from build123d import *

# Parameters (mm, degrees)
SKETCH1_R           = 20
BOSS_EXTRUDE1_DEPTH = 5
BOSS_EXTRUDE2_DEPTH = 4


with BuildPart() as part:
    # Sketch1 → Boss-Extrude1 (new body)
    # profile 1 of 4: a face of its own
    with BuildSketch(Plane.XY):
        with BuildLine():
            Line((0, 14.047165148), (0, 20.609217456))
            add(Edge.make_bspline(
                [(0, 20.609217456), (-5.5, 20.609217456), (-11, 24.303121583)],
                knots=[0.5, 0.5, 0.5, 1, 1, 1], degree=2))
            add(Edge.make_bspline(
                [(-11, 24.303121583), (-25.025952509, 37.034801988), (-53.805838246, 39.750693097), (-64, 20.609217456)],
                knots=[0, 0, 0, 0, 1, 1, 1, 1], degree=3))
            Line((-64, 20.609217456), (-62.236730193, 10.609217456))
            Line((-62.236730193, 10.609217456), (-59.055336952, -7.433360194))
            ThreePointArc((-59.055336952, -7.433360194), (-55.635135519, -13.357322848), (-49.207259422, -15.696878417))
            Line((-49.207259422, -15.696878417), (-31.207259422, -15.696878417))
            ThreePointArc((-31.207259422, -15.696878417), (-26.207259422, -14.357132455), (-22.547005384, -10.696878417))
            Line((-22.547005384, -10.696878417), (-13.886751346, 4.303121583))
            ThreePointArc((-13.886751346, 4.303121583), (-13.219249284, 5.312773474), (-12.434656927, 6.234386612))
            add(Edge.make_bspline(
                [(-12.434656927, 6.234386612), (-6.217328463, 14.047165148), (0, 14.047165148)],
                knots=[0.052283446, 0.052283446, 0.052283446, 0.5, 0.5, 0.5], degree=2))
        make_face()
        with Locations((-38, 9.303121583)):
            Circle(SKETCH1_R, mode=Mode.SUBTRACT)
    # profile 2 of 4: a face of its own
    with BuildSketch(Plane.XY):
        with BuildLine():
            add(Edge.make_bspline(
                [(11, 24.303121583), (5.5, 20.609217456), (0, 20.609217456)],
                knots=[0, 0, 0, 0.5, 0.5, 0.5], degree=2))
            Line((0, 20.609217456), (0, 14.047165148))
            add(Edge.make_bspline(
                [(0, 14.047165148), (6.217328463, 14.047165148), (12.434656927, 6.234386612)],
                knots=[0.5, 0.5, 0.5, 0.947716554, 0.947716554, 0.947716554], degree=2))
            ThreePointArc((12.434656927, 6.234386612), (13.219249284, 5.312773474), (13.886751346, 4.303121583))
            Line((13.886751346, 4.303121583), (22.547005384, -10.696878417))
            ThreePointArc((22.547005384, -10.696878417), (26.207259422, -14.357132455), (31.207259422, -15.696878417))
            Line((31.207259422, -15.696878417), (49.207259422, -15.696878417))
            ThreePointArc((49.207259422, -15.696878417), (55.635135519, -13.357322848), (59.055336952, -7.433360194))
            Line((59.055336952, -7.433360194), (62.236730193, 10.609217456))
            Line((62.236730193, 10.609217456), (64, 20.609217456))
            add(Edge.make_bspline(
                [(11, 24.303121583), (25.025952509, 37.034801988), (53.805838246, 39.750693097), (64, 20.609217456)],
                knots=[0, 0, 0, 0, 1, 1, 1, 1], degree=3))
        make_face()
        with Locations((38, 9.303121583)):
            Circle(SKETCH1_R, mode=Mode.SUBTRACT)
    # profile 3 of 4: a face of its own
    with BuildSketch(Plane.XY):
        Polygon((64, 10.609217456), (64, 20.609217456), (62.236730193, 10.609217456), align=None)
    # profile 4 of 4: a face of its own
    with BuildSketch(Plane.XY):
        Polygon((-62.236730193, 10.609217456), (-64, 20.609217456), (-64, 10.609217456), align=None)
    extrude(amount=BOSS_EXTRUDE1_DEPTH)

    # Sketch3 → Boss-Extrude2 (add)
    with BuildSketch(Plane.ZY.offset(64)):
        with BuildLine():
            Line((5, 20.609217456), (124.102313443, -0.391733869))
            ThreePointArc((124.102313443, -0.391733869), (131.571415965, -2.746732848), (138.176496403, -6.954633166))
            Line((138.176496403, -6.954633166), (153.084888892, -19.464259805))
            ThreePointArc((153.084888892, -19.464259805), (153.968406613, -21.161481556), (153.393030976, -22.986339937))
            Line((153.393030976, -22.986339937), (151.786061952, -24.901451044))
            ThreePointArc((151.786061952, -24.901451044), (150.088840201, -25.784968765), (148.26398182, -25.209593128))
            Line((148.26398182, -25.209593128), (134.895046755, -13.991724646))
            ThreePointArc((134.895046755, -13.991724646), (128.289966317, -9.783824329), (120.820863794, -7.428825349))
            Line((120.820863794, -7.428825349), (5, 12.993517867))
            Line((5, 12.993517867), (5, 10.609217456))
            Line((5, 10.609217456), (0, 10.609217456))
            Line((0, 10.609217456), (0, 20.609217456))
            Line((0, 20.609217456), (5, 20.609217456))
        make_face()
    boss_extrude2 = extrude(amount=-BOSS_EXTRUDE2_DEPTH)

    # Mirror1: Boss-Extrude2 across plane
    add(boss_extrude2.mirror(Plane(origin=(0, 0, 0), x_dir=(0, 0, 1), z_dir=(1, 0, 0))))


solid = part.part
Source: CAD feature listing. Evaluate the final solid. Frame: model axes, mm. A direction names the side the tool comes from. Give positions to 0.01 mm unless a question says otherwise; leave off trailing zeros. Write each loop counter-clockwise with the first axis right and the second up, starting at its lowest first coordinate (ties: lowest second). Pieces come first, ordered by that corner, then holes. Notation, with made-up numbers: (-22.5, 63.25) - (29.5, 63.25) arc R31 ccw to (29.5, 94.25) - close; hole circle Ø2 at (29.25, 31.5). An arc over 180 degrees is marked (long way). Write item = value, one per line. Start each with the question number.
Q1. Pin query (flat end, axial travel): pin 1 Ø0.5 at (x, z) = (63.5, 2) entering from -Y; pin 2 Ø12 at (x, y) = (22.5, 26) entering from +Z; pin 3 Ø2.5 at (x, z) = (-38, 3.5) entering from -Y. Return the tip coordinate at first contact, or that it passes through.
Q2. Reachability of faces 4 (the cylindrical face through (-26.271, -14.394, 2.465)), 5 (the flat face through (60.624, 1.462, 2.465)), 6 (the flat face through (-62.03, 2.64, 63.72)) from +Z, -Z, +X, -X, +Y, -Y: full face, straight path, thin tool, end or side. Return the list, or none.
Q3. Cut plane A-A, the plane z = 132. Return loops of the section in (x, y), then the cut area to 3 significant figures.
Q4. Draft query along X for faces 1 (the cylindrical face through (26.14, -14.32, 2.46)), 2 (the flat face through (62, -13.1, 145.5)), 3 (the flat face through (64, 3, 77)). Return one class per face: +X half, -X half, draft (parallel to the pull), parting line (faces both ways), or undercut.
Q5. Cut plane B-B, the plane z = 67.5. Return loops of the section in (x, y), then the cut area to 3 significant figures.
Q6. Material intervals for probe 1 along Y at (x, z) = (-38, 2.2); probe 2 along X at (y, z) = (19, 13); probe 3 along Z at (x, y) = (55, 26.5), sorted ascending.
Computed values:
q1.pin_1 = 10.61
q1.pin_2 = 5
q1.pin_3 = -15.7
q2.face_4 = +Z, -Z, -Y
q2.face_5 = -Z, +X, -Y
q2.face_6 = +X, -X, -Y
q3.outline = (-64, -11.85) - (-60, -11.85) - (-60, -2.95) - (-64, -2.95) - close; (60, -11.85) - (64, -11.85) - (64, -2.95) - (60, -2.95) - close
q3.area = 71.2 mm²
q4.face_1 = undercut
q4.face_2 = draft
q4.face_3 = +X half
q5.outline = (-64, 1.97) - (-60, 1.97) - (-60, 9.59) - (-64, 9.59) - close; (60, 1.97) - (64, 1.97) - (64, 9.59) - (60, 9.59) - close
q5.area = 60.9 mm²
q6.probe_1 = -15.7 to -10.7, 29.3 to 34.41
q6.probe_2 = -64 to -60, 60 to 64
q6.probe_3 = 0 to 5
